```python
from build123d import *

# Parameters (mm, degrees)
F0_R     = 19.5
F1_DEPTH = 18
F2_R     = 19
F3_DEPTH = 3
F4_R     = 0.75
F5_DEPTH = 7
F6_R     = 1


with BuildPart() as f1:
    # F0 (on Top) → F1 (new body)
    with BuildSketch(Plane.XY):
        Circle(F0_R)
    extrude(amount=F1_DEPTH)

    # F2 (on face) → F3 (cut)
    with BuildSketch(Plane.XY.offset(18)):
        Circle(F2_R)
    extrude(amount=-F3_DEPTH, mode=Mode.SUBTRACT)

    # F4 (on face) → F5 (join)
    with BuildSketch(Plane.XY.offset(15)):
        Circle(F4_R)
    extrude(amount=F5_DEPTH)

    # F6
    f6_edges = [f1.edges().sort_by_distance(p)[0] for p in [
        (-19.5, 0, 0),
    ]]
    fillet(f6_edges, radius=F6_R)


solid = f1.part
```
The listing builds one solid part. Answer for the finished solid, in the listing's coordinates (mm). A direction names the side the tool comes from. Coordinates: 2 decimals unless noted, no trailing zeros. Loops run counter-clockwise (first coordinate to the right, second up) from the corner with the lowest first, then second, coordinate; pieces in that order, holes last. Notation, with made-up numbers: (45, 80.25) -> (89, 80.25) arc R5 cw to (89, 86.25) -> close; hole circle Ø11 at (-6.75, 9.25). An arc over 180 degrees is marked (long way). Use one line per item in the form item = value. Start each with the question number.
Item 1: The mould has two halves that part along Y. Classify faces 1 (the face through (-0.75, 0.03, 18.45)), 2 (the face through (0, 0, 0)), 3 (the face through (-2.539, 19.334, 9.381)): released by +Y, released by -Y, zero draft, split by the parting line, or undercut.
Item 2: The part is cut by section D-D on z = 9.75. Determine the outline of the cut face in (x, y).
Item 3: The part is cut by section B-B on z = 16.5. Determine the outline of the cut face in (x, y).
Item 4: Consider L1, parallel to Y at x = 0, z = 16.8; L2, parallel to Z at x = 14.5, y = -11; L3, parallel to Y at x = -2, z = 16. Determine where each line is inside the solid, lowest interval first. Write a range as [from, to].
Item 5: The part is cut by section A-A on y = 0. Determine the outline of the cut face in (x, z), then the cut area to 3 significant figures.
Item 6: A tool of negligible diameter and unlimited length cuts with its end or side. For faces 4 (the face through (0, 0, 22)), 5 (the face through (0, -4, 15)), from which of +Z, -Z, +X, -X, +Y, -Y can it reach the whole face along a straight path? Write none if from no direction.
Item 7: Flat-ended cylindrical pins translate along their axes: pin 1 Ø5 at (y, z) = (-9.5, 10) entering from +X; pin 2 Ø8 at (x, z) = (-15, 11.5) entering from +Y; pin 3 Ø1.5 at (y, z) = (14.5, 17.5) entering from +X. Find the tip coordinate at first contact, or state that the pin passes through.
Answer key:
q1.face_1 = undercut
q1.face_2 = zero draft
q1.face_3 = split by the parting line
q2.outline = circle Ø39 at (0, 0)
q3.outline = circle Ø39 at (0, 0); circle Ø1.5 at (0, 0); hole circle Ø38 at (0, 0)
q4.L1 = [-19.5, -19], [-0.75, 0.75], [19, 19.5]
q4.L2 = [0, 15]
q4.L3 = [-19.4, -18.89], [18.89, 19.4]
q5.outline = (-19.5, 1) arc R1 ccw to (-18.5, 0) -> (18.5, 0) arc R1 ccw to (19.5, 1) -> (19.5, 18) -> (19, 18) -> (19, 15) -> (0.75, 15) -> (0.75, 22) -> (-0.75, 22) -> (-0.75, 15) -> (-19, 15) -> (-19, 18) -> (-19.5, 18) -> close
q5.area = 598 mm2
q6.face_4 = +Z, +X, -X, +Y, -Y
q6.face_5 = +Z
q7.pin_1 = 18.2
q7.pin_2 = 16.1
q7.pin_3 = 13.83
